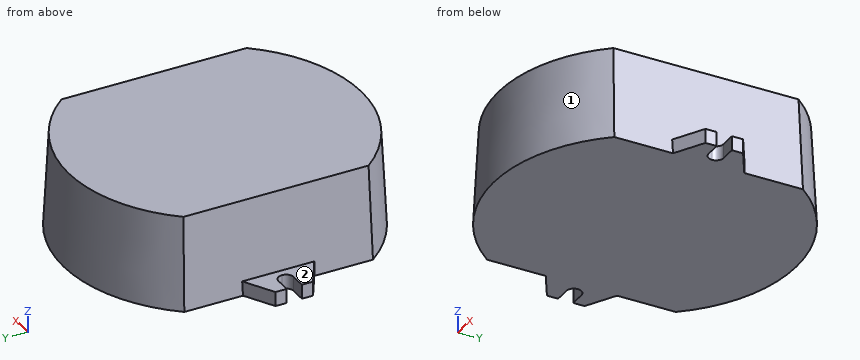
```python
from build123d import *

# Parameters (mm, degrees)
F0_R     = 40
F1_DEPTH = 25
F1_TAPER = 3
F2_W     = 25.4
F2_H     = 101.6
F3_DEPTH = 25.001
F3_TAPER = 3
F5_DEPTH = 3.81


with BuildPart() as f1:
    # F0 (on Top) → F1 (new body)
    with BuildSketch(Plane.XY):
        Circle(F0_R)
    extrude(amount=F1_DEPTH, taper=F1_TAPER)

    # F2 (on face) → F3 (cut, through all)
    with BuildSketch(Plane.XY.offset(25)):
        with Locations((-42.7, 0)):
            Rectangle(F2_W, F2_H)
        with Locations((42.7, 0)):
            Rectangle(F2_W, F2_H)
    extrude(amount=-F3_DEPTH, taper=F3_TAPER, mode=Mode.SUBTRACT)

    # F4 (on face) → F5 (join)
    with BuildSketch(Plane(origin=(0, 0, 0), x_dir=(1, 0, 0), z_dir=(0, 0, -1))):
        with BuildLine():
            ThreePointArc((-35, 2), (-33.5857864376, 1.4142135624), (-33, 0))
            ThreePointArc((-33, 0), (-33.5857864376, -1.4142135624), (-35, -2))
            Line((-35, -2), (-39, -2))
            Line((-39, -2), (-39, -4.9638475773))
            Line((-39, -4.9638475773), (-30, -10.16))
            Line((-30, -10.16), (-30, 10.16))
            Line((-30, 10.16), (-39, 4.9638475773))
            Line((-39, 4.9638475773), (-39, 2))
            Line((-39, 2), (-35, 2))
        make_face()
        with BuildLine():
            ThreePointArc((33, 0), (33.5857864376, 1.4142135624), (35, 2))
            Line((35, 2), (39, 2))
            Line((39, 2), (39, 4.9638475773))
            Line((39, 4.9638475773), (30, 10.16))
            Line((30, 10.16), (30, -10.16))
            Line((30, -10.16), (39, -4.9638475773))
            Line((39, -4.9638475773), (39, -2))
            Line((39, -2), (35, -2))
            ThreePointArc((35, -2), (33.5857864376, -1.4142135624), (33, 0))
        make_face()
    extrude(amount=-F5_DEPTH)


solid = f1.part
```
Source: CAD feature listing. Evaluate the final solid. Frame: model axes, mm. Face numbers are marked on the shaded views. A direction names the side the tool comes from. Round coordinates to 2 decimals unless told otherwise and drop trailing zeros. One line per item, written item: value. Start each with the question number.
Q1. Access query for the marked faces 1 and 2. Directions: +Z, -Z, +X, -X, +Y, -Y. A direction counts if a zero-diameter tool reaches every point of the face in a straight line with its end or side. Return the directions, or none.
Q2. Material intervals for probe 1 along Y at (x, z) = (-24.5, 7.5); probe 2 along X at (y, z) = (-10, 2.75); probe 3 along X at (y, z) = (-9.5, 20.25), sorted ascending.
Q3. Pin query (flat end, axial travel): pin 1 (1.1 mm diameter, centred on x = -37.5, z = 2, fed in from -Y); pin 2 (1 mm diameter, centred on x = 16.5, z = 20.5, fed in from +Y); pin 3 (1.9 mm diameter, centred on x = 37, z = 1.5, fed in from -Y). Return the tip coordinate at first contact, or that it passes through.
Findings below:
1. face 1: +Z, -Y
1. face 2: +Z, -X, +Y, -Y
2. probe 1: -31.12 to 31.12
2. probe 2: -31.17 to 31.17
2. probe 3: -30.25 to 30.25
3. pin 1: y = -6.15
3. pin 2: y = 35.49
3. pin 3: y = -6.67
